Source: CAD feature listing. Evaluate the final solid. Frame: model axes, mm. A direction names the side the tool comes from. Give positions to 0.01 mm unless a question says otherwise; leave off trailing zeros. Order: outer loops, then holes, each group sorted by start corner. A loop starts at its lowest first (then second) coordinate and runs counter-clockwise, first axis right, second up. Notation, with made-up numbers: M 65.5,84 L 83.5,84 A18 ccw 83.5,109 Z; hole C -39,45.25 d2. An arc over 180 degrees is marked long. Answer in a Markdown table with one row per item. Add a question column.
(1) Set-up query: faces 1 (the face through (-7, 4.762, -5)), 2 (the face through (525.018, 3, 56)). Return all of +Z, -Z, +X, -X, +Y, -Y with unobstructed straight access to the full face (end or side cutting, diameter ignored); none if empty.
(2) Pin query (flat end, axial travel): P1, Ø12, axis at x = -189.5, y = 28, coming from the +Z side; P2, Ø8, axis at x = 382.5, y = 102.5, coming from the +Z side; P3, Ø10, axis at x = 412, y = 75.5, coming from the -Z side. Return the tip coordinate at first contact, or that it passes through.
(3) Section query A-A, the plane x = -16.5. Return loops of the section in (y, z), plus the area to 3 significant figures.
(4) Section query C-C, the plane y = 115. Return loops of the section in (x, z).
(5) Material intervals for line 1 along Y through (x, z) = (-373, 39); line 2 along Z through (x, y) = (419, 30); line 3 along Z through (x, y) = (-200, 79), sorted ascending.
(6) Section query B-B, the plane z = -149. Return loops of the section in (x, y).
from build123d import *

# Parameters (mm, degrees)
SKETCH1_W           = 1050.036
SKETCH1_H           = 457.2
BOSS_EXTRUDE1_DEPTH = 4.7625
BOSS_EXTRUDE2_DEPTH = 1050.036
SKETCH9_R           = 1.5875
CUT_EXTRUDE3_DEPTH  = 574.601708141
CIRPATTERN1_COUNT   = 2
CIRPATTERN1_ANGLE   = 120
CUT_EXTRUDE2_REACH  = 826.59
SKETCH8_W           = 1050.036
SKETCH8_H           = 311.15
FILLET1_R           = 2.38125


with BuildPart() as part:
    # Sketch1 → Boss-Extrude1 (new body)
    with BuildSketch(Plane(origin=(0, 0, 0), x_dir=(1, 0, 0), z_dir=(0, 1, 0))):
        Rectangle(SKETCH1_W, SKETCH1_H)
    boss_extrude1 = extrude(amount=BOSS_EXTRUDE1_DEPTH)

    # Sketch2 → Boss-Extrude2 (add)
    with BuildSketch(Plane.ZY.offset(525.018)):
        with BuildLine():
            Line((228.6, 4.7625), (228.6, 0))
            ThreePointArc((228.6, 0), (230.98125, 2.38125), (228.6, 4.7625))
        make_face()
    extrude(amount=-BOSS_EXTRUDE2_DEPTH)

    # Sketch9 → Cut-Extrude3 (cut, through all)
    with BuildSketch(Plane(origin=(0, 4.7625, 0), x_dir=(1, 0, 0), z_dir=(0, 1, 0))):
        with Locations(Location((520.2555, -210.3923148, 0), (0, 0, 270))):
            Circle(SKETCH9_R)
        with Locations(Location((-520.2555, -210.3923148, 0), (0, 0, 270))):
            Circle(SKETCH9_R)
    cut_extrude3 = extrude(amount=-CUT_EXTRUDE3_DEPTH, mode=Mode.SUBTRACT)

    # CirPattern1: Boss-Extrude1, Cut-Extrude3 ×2 about axis
    cirpattern1_axis = Axis((0, 2.38125, 228.6), (1, 0, 0))
    add([boss_extrude1.rotate(cirpattern1_axis, i * CIRPATTERN1_ANGLE / (CIRPATTERN1_COUNT - 1)) for i in range(1, CIRPATTERN1_COUNT)])
    add([cut_extrude3.rotate(cirpattern1_axis, i * CIRPATTERN1_ANGLE / (CIRPATTERN1_COUNT - 1)) for i in range(1, CIRPATTERN1_COUNT)], mode=Mode.SUBTRACT)

    # Sketch8 → Cut-Extrude2 (cut, up to next)
    with BuildSketch(Plane(origin=(0, -97.200766153, 168.356665511), x_dir=(-1, 0, 0), z_dir=(0, 0.500000000000004, -0.8660254037844365)), mode=Mode.PRIVATE) as cut_extrude2_sk1:
        with Locations((0, 417.987222993)):
            Rectangle(SKETCH8_W, SKETCH8_H)
    cut_extrude2_tool1 = extrude(cut_extrude2_sk1.sketch, amount=-CUT_EXTRUDE2_REACH, mode=Mode.PRIVATE) & part.part
    add(cut_extrude2_tool1.solids().sort_by_distance((0, 264.786787, 377.350277))[0], mode=Mode.SUBTRACT)

    # Fillet1
    fillet1_edges = [part.edges().sort_by_distance(p)[0] for p in [
        (0, 4.7625, 227.225184671),
    ]]
    fillet(fillet1_edges, radius=FILLET1_R)


solid = part.part
Values follow:
| question | item | result |
|---|---|---|
| 1 | face 1 | -Z, +X, -X, +Y |
| 1 | face 2 | +Z, -Z, +X, +Y, -Y |
| 2 | P1 | stops at z = 249.6 |
| 2 | P2 | stops at z = 291.46 |
| 2 | P3 | stops at z = 265.18 |
| 3 | outline | M 0,-228.6 L 4.76,-228.6 L 4.76,225.85 A2.38 cw 5.95,227.91 L 130.05,299.56 L 127.67,303.69 L 1.19,230.66 A2.38 ccw 0,228.6 Z |
| 3 | area | 2,870 mm² |
| 4 | outline | M -525.02,290.87 L 525.02,290.87 L 525.02,296.37 L -525.02,296.37 Z |
| 5 | line 1 | y = 0 to 4.76 |
| 5 | line 2 | z = 241.8 to 247.3 |
| 5 | line 3 | z = 270.09 to 275.59 |
| 6 | outline | M -525.02,0 L 525.02,0 L 525.02,4.76 L -525.02,4.76 Z |
